from build123d import *

# Parameters (mm, degrees)
BOSS_EXTRUDE2_DEPTH     = 9
SKETCH4_W               = 5
SKETCH4_H               = 1
BOSS_EXTRUDE3_DEPTH     = 5
SKETCH5_R               = 1
CUT_EXTRUDE1_DEPTH      = 5
FILLET1_R               = 1
FILLET2_R               = 1
FILLET3_R               = 3
FILLET4_R               = 3
BOSS_EXTRUDE4_DEPTH     = 12
FILLET6_R               = 0.25
SKETCH10_R              = 1.5
CUT_EXTRUDE7_DEPTH      = 44.13930922
CUT_EXTRUDE7_DEPTH_BACK = 44.13930922
SKETCH12_R              = 0.75
CUT_EXTRUDE8_DEPTH      = 3
SKETCH13_W              = 1
SKETCH13_H              = 5
BOSS_EXTRUDE5_DEPTH     = 2
SKETCH14_W              = 5
SKETCH14_H              = 1
BOSS_EXTRUDE6_DEPTH     = 1
FILLET7_R               = 0.5
FILLET8_R               = 0.5
FILLET9_R               = 0.5
CUT_EXTRUDE9_DEPTH      = 10
BOSS_EXTRUDE7_DEPTH     = 1
SKETCH18_R              = 1.5
CUT_EXTRUDE12_DEPTH     = 44.358966777
SKETCH19_R              = 0.75
CUT_EXTRUDE14_DEPTH     = 44.358966777
SKETCH20_R              = 2
BOSS_EXTRUDE8_DEPTH     = 1.5
FILLET10_R              = 0.25
SKETCH21_R              = 2.5
CUT_EXTRUDE15_DEPTH     = 5
SKETCH22_R              = 3
SKETCH22_R_2            = 2.5
BOSS_EXTRUDE9_DEPTH     = 0.25
SKETCH24_R              = 2
CUT_EXTRUDE16_DEPTH     = 2
SKETCH25_R              = 1
CUT_EXTRUDE17_DEPTH     = 5


with BuildPart() as part:
    # Sketch2 → Boss-Extrude2 (new body)
    with BuildSketch(Plane(origin=(0, 0, 0), x_dir=(1, 0, 0), z_dir=(0, 1, 0))):
        Polygon((0, 11), (31, 11), (31, 13.5), (31, 22), (0, 22), align=None)
        Polygon((31, 8.5), (31, 11), (0, 11), (0, 0), (31, 0), align=None)
    extrude(amount=BOSS_EXTRUDE2_DEPTH)

    # Sketch4 → Boss-Extrude3 (add)
    with BuildSketch(Plane(origin=(31, 0, 0), x_dir=(0, 0, -1), z_dir=(1, 0, 0))):
        with Locations((11, 0.5)):
            Rectangle(SKETCH4_W, SKETCH4_H)
    extrude(amount=BOSS_EXTRUDE3_DEPTH)

    # Sketch5 → Cut-Extrude1 (cut)
    with BuildSketch(Plane(origin=(0, 1, 0), x_dir=(1, 0, 0), z_dir=(0, 1, 0))):
        with Locations(Location((33.5, 11, 0), (0, 0, 270))):
            Circle(SKETCH5_R)
    extrude(amount=-CUT_EXTRUDE1_DEPTH, mode=Mode.SUBTRACT)

    # Fillet1
    fillet1_edges = [part.edges().sort_by_distance(p)[0] for p in [
        (31, 0.5, -8.5),
    ]]
    fillet(fillet1_edges, radius=FILLET1_R)

    # Fillet2
    fillet2_edges = [part.edges().sort_by_distance(p)[0] for p in [
        (31, 0.5, -13.5),
    ]]
    fillet(fillet2_edges, radius=FILLET2_R)

    # Fillet3
    fillet3_edges = [part.edges().sort_by_distance(p)[0] for p in [
        (31, 4.5, 0),
    ]]
    fillet(fillet3_edges, radius=FILLET3_R)

    # Fillet4
    fillet4_edges = [part.edges().sort_by_distance(p)[0] for p in [
        (31, 4.5, -22),
    ]]
    fillet(fillet4_edges, radius=FILLET4_R)

    # Sketch6 → Boss-Extrude4 (add)
    with BuildSketch(Plane.ZY):
        with BuildLine():
            Line((-22, 0), (-11, 0))
            Line((-11, 0), (-11, 9))
            Line((-11, 9), (-19, 9))
            ThreePointArc((-19, 9), (-21.121122912, 5.415884648), (-22, 1.344936316))
            Line((-22, 1.344936316), (-22, 0))
        make_face()
        with BuildLine():
            Line((-11, 9), (-11, 0))
            Line((-11, 0), (0, 0))
            Line((0, 0), (0, 1.344936316))
            ThreePointArc((0, 1.344936316), (-0.878877088, 5.415884648), (-3, 9))
            Line((-3, 9), (-11, 9))
        make_face()
    extrude(amount=BOSS_EXTRUDE4_DEPTH)

    # Fillet6
    fillet6_edges = [part.edges().sort_by_distance(p)[0] for p in [
        (36, 0.5, -13.5),
        (36, 0.5, -8.5),
    ]]
    fillet(fillet6_edges, radius=FILLET6_R)

    # Sketch10 → Cut-Extrude7 (cut, two sides)
    with BuildSketch(Plane(origin=(0, 9, 0), x_dir=(1, 0, 0), z_dir=(0, 1, 0))) as cut_extrude7_sk:
        with Locations(Location((5, 19.5, 0), (0, 0, 270))):
            Circle(SKETCH10_R)
        with Locations(Location((5, 2.5, 0), (0, 0, 270))):
            Circle(SKETCH10_R)
    extrude(amount=CUT_EXTRUDE7_DEPTH, mode=Mode.SUBTRACT)
    extrude(cut_extrude7_sk.sketch, amount=-CUT_EXTRUDE7_DEPTH_BACK, mode=Mode.SUBTRACT)

    # Sketch12 → Cut-Extrude8 (cut)
    with BuildSketch(Plane(origin=(0, 9, 0), x_dir=(1, 0, 0), z_dir=(0, 1, 0))):
        with Locations(Location((2, 2, 0), (0, 0, 270))):
            Circle(SKETCH12_R)
        with Locations(Location((2, 20, 0), (0, 0, 270))):
            Circle(SKETCH12_R)
    extrude(amount=-CUT_EXTRUDE8_DEPTH, mode=Mode.SUBTRACT)

    # Sketch13 → Boss-Extrude5 (add)
    with BuildSketch(Plane(origin=(0, 9, 0), x_dir=(1, 0, 0), z_dir=(0, 1, 0))):
        with Locations((-7.5, 11)):
            Rectangle(SKETCH13_W, SKETCH13_H)
    extrude(amount=BOSS_EXTRUDE5_DEPTH)

    # Sketch14 → Boss-Extrude6 (add)
    with BuildSketch(Plane(origin=(-7, 0, 0), x_dir=(0, 0, -1), z_dir=(1, 0, 0))):
        with Locations((11, 10.5)):
            Rectangle(SKETCH14_W, SKETCH14_H)
    extrude(amount=BOSS_EXTRUDE6_DEPTH)

    # Fillet7
    fillet7_edges = [part.edges().sort_by_distance(p)[0] for p in [
        (-8, 11, -11),
    ]]
    fillet(fillet7_edges, radius=FILLET7_R)

    # Fillet8
    fillet8_edges = [part.edges().sort_by_distance(p)[0] for p in [
        (-8, 9, -11),
    ]]
    fillet(fillet8_edges, radius=FILLET8_R)

    # Fillet9
    fillet9_edges = [part.edges().sort_by_distance(p)[0] for p in [
        (-6, 11, -11),
    ]]
    fillet(fillet9_edges, radius=FILLET9_R)

    # Sketch16 → Cut-Extrude9 (cut)
    with BuildSketch(Plane.ZY.offset(12)):
        with BuildLine():
            Line((-18.232108037, 8.359420628), (-3.767891963, 8.359420628))
            ThreePointArc((-3.767891963, 8.359420628), (-1.809932353, 5.051006457), (-0.998661194, 1.293207997))
            Line((-0.998661194, 1.293207997), (-0.998661194, 0))
            Line((-0.998661194, 0), (-21, 0))
            Line((-21, 0), (-21.001338806, 1.293207997))
            ThreePointArc((-21.001338806, 1.293207997), (-20.190067647, 5.051006457), (-18.232108037, 8.359420628))
        make_face()
    extrude(amount=-CUT_EXTRUDE9_DEPTH, mode=Mode.SUBTRACT)

    # Sketch17 → Boss-Extrude7 (add)
    with BuildSketch(Plane(origin=(0, 9, 0), x_dir=(1, 0, 0), z_dir=(0, 1, 0))):
        with BuildLine():
            Line((0, 3), (0, 19))
            Line((0, 19), (0, 22))
            Line((0, 22), (28, 22))
            ThreePointArc((28, 22), (30.121320344, 21.121320344), (31, 19))
            Line((31, 19), (31, 3))
            ThreePointArc((31, 3), (30.121320344, 0.878679656), (28, 0))
            Line((28, 0), (0, 0))
            Line((0, 0), (0, 3))
        make_face()
    extrude(amount=BOSS_EXTRUDE7_DEPTH)

    # Sketch18 → Cut-Extrude12 (cut, through all)
    with BuildSketch(Plane(origin=(0, 10, 0), x_dir=(1, 0, 0), z_dir=(0, 1, 0))):
        with Locations(Location((5, 19.5, 0), (0, 0, 270))):
            Circle(SKETCH18_R)
        with Locations(Location((5, 2.5, 0), (0, 0, 270))):
            Circle(SKETCH18_R)
    extrude(amount=-CUT_EXTRUDE12_DEPTH, mode=Mode.SUBTRACT)

    # Sketch19 → Cut-Extrude14 (cut, through all)
    with BuildSketch(Plane(origin=(0, 10, 0), x_dir=(1, 0, 0), z_dir=(0, 1, 0))):
        with Locations(Location((2, 20, 0), (0, 0, 270))):
            Circle(SKETCH19_R)
        with Locations(Location((2, 2, 0), (0, 0, 270))):
            Circle(SKETCH19_R)
    extrude(amount=-CUT_EXTRUDE14_DEPTH, mode=Mode.SUBTRACT)

    # Sketch20 → Boss-Extrude8 (add)
    with BuildSketch(Plane(origin=(0, 10, 0), x_dir=(1, 0, 0), z_dir=(0, 1, 0))):
        with Locations(Location((9, 11, 0), (0, 0, 270))):
            Circle(SKETCH20_R)
    extrude(amount=BOSS_EXTRUDE8_DEPTH)

    # Fillet10
    fillet10_edges = [part.edges().sort_by_distance(p)[0] for p in [
        (9, 11.5, -13),
    ]]
    fillet(fillet10_edges, radius=FILLET10_R)

    # Sketch21 → Cut-Extrude15 (cut)
    with BuildSketch(Plane(origin=(0, 10, 0), x_dir=(1, 0, 0), z_dir=(0, 1, 0))):
        with Locations(Location((20, 11, 0), (0, 0, 270))):
            Circle(SKETCH21_R)
    extrude(amount=-CUT_EXTRUDE15_DEPTH, mode=Mode.SUBTRACT)

    # Sketch22 → Boss-Extrude9 (add)
    with BuildSketch(Plane(origin=(0, 10, 0), x_dir=(1, 0, 0), z_dir=(0, 1, 0))):
        with Locations(Location((20, 11, 0), (0, 0, 270))):
            Circle(SKETCH22_R)
        with Locations(Location((20, 11, 0), (0, 0, 270))):
            Circle(SKETCH22_R_2, mode=Mode.SUBTRACT)
    extrude(amount=BOSS_EXTRUDE9_DEPTH)

    # Sketch24 → Cut-Extrude16 (cut)
    with BuildSketch(Plane(origin=(0, 10, 0), x_dir=(1, 0, 0), z_dir=(0, 1, 0))):
        with Locations((2.5, 17.5)):
            Circle(SKETCH24_R)
        with Locations((2.5, 4.5)):
            Circle(SKETCH24_R)
    extrude(amount=-CUT_EXTRUDE16_DEPTH, mode=Mode.SUBTRACT)

    # Sketch25 → Cut-Extrude17 (cut)
    with BuildSketch(Plane(origin=(0, 10, 0), x_dir=(1, 0, 0), z_dir=(0, 1, 0))):
        with Locations(Location((2.5, 17.5, 0), (0, 0, 270))):
            Circle(SKETCH25_R)
        with Locations(Location((2.5, 4.5, 0), (0, 0, 270))):
            Circle(SKETCH25_R)
    extrude(amount=-CUT_EXTRUDE17_DEPTH, mode=Mode.SUBTRACT)


solid = part.part
Could you check a few things on this model? Use its own coordinates, in mm. A direction names the side the tool comes from. Round coordinates to 2 decimals unless told otherwise and drop trailing zeros. Order: outer loops, then holes, each group sorted by start corner. A loop starts at its lowest first (then second) coordinate and runs counter-clockwise, first axis right, second up.
(1) Imagine slicing it at B-B (z = -7). Write out the boundary of the cut face in (x, y), plus the area to 3 significant figures.
Response values:
outline: (-12, 8.36) - (-2, 8.36) - (-2, 0) - (31, 0) - (31, 10) - (0, 10) - (0, 9) - (-12, 9) - close
area: 334 mm2
(2) Which directions (+Z, -Z, +X, -X, +Y, -Y) give clear straight access to the entire face, cutting with the end or side of a thin tool? Please do faces 1 (the flat face through (20, 5, -11)), 2 (the flat face through (22, 10.25, -13)), 3 (the flat face through (-7, 8.359, -11)), 4 (the flat face through (-7, 11, -11)).
Response values:
face 1: +Y
face 2: +Z, -Z, +X, +Y
face 3: -X, -Y
face 4: +Z, -Z, -X, +Y
(3) Imagine slicing it at C-C (y = 6.75). Write out the boundary of the cut face in (x, z).
Response values:
outline: (-12, -20.51) - (0, -20.51) - (0, -22) - (28, -22) arc R3 ccw to (31, -19) - (31, -3) arc R3 ccw to (28, 0) - (0, 0) - (0, -1.49) - (-12, -1.49) - (-12, -2.64) - (-2, -2.64) - (-2, -19.36) - (-12, -19.36) - close; hole circle Ø1.5 at (2, -20); hole circle Ø1.5 at (2, -2); hole circle Ø2 at (2.5, -17.5); hole circle Ø2 at (2.5, -4.5); hole circle Ø3 at (5, -19.5); hole circle Ø3 at (5, -2.5); hole circle Ø5 at (20, -11)
(4) Please list where these lines run through material, in increasing order: line 1 along Z through (x, y) = (5, 6.5); line 2 along X through (y, z) = (7.1, -17.5); line 3 along Z through (x, y) = (2.5, 9.1).
Response values:
line 1: z = -22 to -21, -18 to -4, -1 to 0
line 2: x = -2 to 1.5, 3.5 to 31
line 3: z = -22 to -20.56, -15.5 to -6.5, -1.44 to 0
(5) If we mould it in two halves opening along Z, with no side actions, what happens to faces 5 (the flat face through (33.8, 0.5, -8.5)), 6 (the flat face through (9, 11.5, -11)), 7 (the cylindrical face through (6.01, 5.07, -20.61))? For each: released by +Z, released by -Z, zero draft, split by the parting line, or undercut.
Response values:
face 5: released by +Z
face 6: zero draft
face 7: undercut
(6) I'm going to push flat-ended pins straight in: pin 1 (3 mm diameter, centred on y = 8, z = -11, fed in from +X); pin 2 (2 mm diameter, centred on x = 11, z = -14.5, fed in from -Y); pin 3 (9.5 mm diameter, centred on x = -4, z = -9, fed in from +Y); pin 4 (5.5 mm diameter, centred on x = 34.5, z = -12, fed in from +Y). Where does each tip first touch, or does it pass through?
Response values:
pin 1: stops at x = 31
pin 2: stops at y = 0
pin 3: stops at y = 11
pin 4: stops at y = 1
(7) Imagine slicing it at D-D (z = -2). Write out the boundary of the cut face in (x, y), plus the area to 3 significant figures.
Response values:
outline: (-12, 5.51) - (-2, 5.51) - (-2, 0) - (1.25, 0) - (1.25, 10) - (0, 10) - (0, 7.63) - (-12, 7.63) - close; (2.75, 0) - (3.59, 0) - (3.59, 10) - (2.75, 10) - close; (6.41, 0) - (30.83, 0) - (30.83, 10) - (6.41, 10) - close
area: 301 mm2
(8) Imagine slicing it at A-A (x = 5). Write out the boundary of the cut face in (y, z), plus the area to 3 significant figures.
Response values:
outline: (0, -22) - (10, -22) - (10, -21) - (0, -21) - close; (0, -18) - (10, -18) - (10, -4) - (0, -4) - close; (0, -1) - (10, -1) - (10, 0) - (0, 0) - close
area: 160 mm2
